from build123d import *

# Parameters (mm, degrees)
SKETCH1_W                    = 42.3
SKETCH1_H                    = 42.3
BOSS_EXTRUDE1_DEPTH          = 48
SKETCH2_R                    = 11
BOSS_EXTRUDE2_DEPTH          = 2
SKETCH3_R                    = 2.5
BOSS_EXTRUDE3_DEPTH          = 23
FILLET2_R                    = 0.3
CHAMFER1_SIZE                = 0.5
SKETCH4_R                    = 1.5
CUT_EXTRUDE1_DEPTH           = 4.5
CHAMFER2_SIZE                = 0.3
CUT_EXTRUDE2_START           = -0.5
SKETCH5_R                    = 16.5
SKETCH5_R_2                  = 11
CUT_EXTRUDE2_DEPTH           = 0.5
CUT_EXTRUDE_THIN1_DEPTH      = 57.556564606
CUT_EXTRUDE_THIN1_DEPTH_BACK = 57.556564606
SKETCH7_R                    = 3.5
SKETCH7_R_2                  = 3
CUT_EXTRUDE3_DEPTH           = 5
SKETCH8_W                    = 8
SKETCH8_H                    = 5
BOSS_EXTRUDE4_DEPTH          = 2
FILLET3_R                    = 1


with BuildPart() as part:
    # Sketch1 → Boss-Extrude1 (new body)
    with BuildSketch(Plane(origin=(0, 0, 0), x_dir=(1, 0, 0), z_dir=(0, 1, 0))):
        Rectangle(SKETCH1_W, SKETCH1_H)
    extrude(amount=BOSS_EXTRUDE1_DEPTH)

    # Sketch2 → Boss-Extrude2 (add)
    with BuildSketch(Plane(origin=(0, 48, 0), x_dir=(1, 0, 0), z_dir=(0, 1, 0))):
        with Locations(Location((0, 0, 0), (0, 0, 90))):
            Circle(SKETCH2_R)
    extrude(amount=BOSS_EXTRUDE2_DEPTH)

    # Sketch3 → Boss-Extrude3 (add)
    with BuildSketch(Plane(origin=(0, 50, 0), x_dir=(1, 0, 0), z_dir=(0, 1, 0))):
        with Locations(Location((0, 0, 0), (0, 0, 270))):
            Circle(SKETCH3_R)
    extrude(amount=BOSS_EXTRUDE3_DEPTH)

    # Fillet2
    fillet2_edges = [part.edges().sort_by_distance(p)[0] for p in [
        (0, 50, 11),
    ]]
    fillet(fillet2_edges, radius=FILLET2_R)

    # Chamfer1
    chamfer1_edges = [part.edges().sort_by_distance(p)[0] for p in [
        (0, 73, -2.5),
    ]]
    chamfer(chamfer1_edges, length=CHAMFER1_SIZE)

    # Sketch4 → Cut-Extrude1 (cut)
    with BuildSketch(Plane(origin=(0, 48, 0), x_dir=(1, 0, 0), z_dir=(0, 1, 0))):
        with Locations(Location((-15.5, -15.5, 0), (0, 0, 270))):
            Circle(SKETCH4_R)
        with Locations(Location((15.5, -15.5, 0), (0, 0, 270))):
            Circle(SKETCH4_R)
        with Locations(Location((15.5, 15.5, 0), (0, 0, 270))):
            Circle(SKETCH4_R)
        with Locations(Location((-15.5, 15.5, 0), (0, 0, 270))):
            Circle(SKETCH4_R)
    extrude(amount=-CUT_EXTRUDE1_DEPTH, mode=Mode.SUBTRACT)

    # Chamfer2
    chamfer2_edges = [part.edges().sort_by_distance(p)[0] for p in [
        (-15.5, 48, 14),
        (15.5, 48, 14),
        (15.5, 48, -17),
        (-15.5, 48, -17),
    ]]
    chamfer(chamfer2_edges, length=CHAMFER2_SIZE)

    # Sketch5 → Cut-Extrude2 (cut)
    with BuildSketch(Plane(origin=(0, 48, 0), x_dir=(1, 0, 0), z_dir=(0, 1, 0)).offset(CUT_EXTRUDE2_START)):
        with Locations(Location((0, 0, 0), (0, 0, 270))):
            Circle(SKETCH5_R)
        with Locations(Location((0, 0, 0), (0, 0, 270))):
            Circle(SKETCH5_R_2, mode=Mode.SUBTRACT)
    extrude(amount=CUT_EXTRUDE2_DEPTH, mode=Mode.SUBTRACT)

    # Sketch6 → Cut-Extrude-Thin1 (cut, two sides: drawn at the far end of the back side and taken through both)
    with BuildSketch(Plane(origin=(0, 48, 0), x_dir=(1, 0, 0), z_dir=(0, 1, 0)).offset(-CUT_EXTRUDE_THIN1_DEPTH_BACK)):
        Polygon((-21.15, -17.15), (-17.15, -21.15), (-24.221067812, -28.221067812), (-28.221067812, -24.221067812), align=None)
        Polygon((17.15, -21.15), (21.15, -17.15), (28.221067812, -24.221067812), (24.221067812, -28.221067812), align=None)
        Polygon((21.15, 17.15), (17.15, 21.15), (24.221067812, 28.221067812), (28.221067812, 24.221067812), align=None)
        Polygon((-17.15, 21.15), (-21.15, 17.15), (-28.221067812, 24.221067812), (-24.221067812, 28.221067812), align=None)
    extrude(amount=CUT_EXTRUDE_THIN1_DEPTH + CUT_EXTRUDE_THIN1_DEPTH_BACK, mode=Mode.SUBTRACT)

    # Sketch7 → Cut-Extrude3 (cut)
    with BuildSketch(Plane.XZ):
        with Locations(Location((0, 0, 0), (0, 0, 270))):
            Circle(SKETCH7_R)
        with Locations(Location((-15.5, 15.5, 0), (0, 0, 270))):
            Circle(SKETCH7_R_2)
        with Locations(Location((15.5, 15.5, 0), (0, 0, 270))):
            Circle(SKETCH7_R_2)
        with Locations(Location((15.5, -15.5, 0), (0, 0, 270))):
            Circle(SKETCH7_R_2)
        with Locations(Location((-15.5, -15.5, 0), (0, 0, 270))):
            Circle(SKETCH7_R_2)
    extrude(amount=-CUT_EXTRUDE3_DEPTH, mode=Mode.SUBTRACT)

    # Sketch8 → Boss-Extrude4 (add)
    with BuildSketch(Plane.ZY.offset(21.15)):
        with Locations((0, 5)):
            Rectangle(SKETCH8_W, SKETCH8_H)
    extrude(amount=BOSS_EXTRUDE4_DEPTH)

    # Fillet3
    fillet3_edges = [part.edges().sort_by_distance(p)[0] for p in [
        (-23.15, 5, 4),
        (-23.15, 7.5, 0),
        (-23.15, 5, -4),
        (-23.15, 2.5, 0),
    ]]
    fillet(fillet3_edges, radius=FILLET3_R)


solid = part.part
Can you work these out from the model? Positions are in its coordinate system, mm. A direction names the side the tool comes from. Give positions to 0.01 mm unless a question says otherwise; leave off trailing zeros. Write each loop counter-clockwise with the first axis right and the second up, starting at its lowest first coordinate (ties: lowest second). Pieces come first, ordered by that corner, then holes. Notation, with made-up numbers: (62.25, 39) -> (68.25, 39) arc R9 ccw to (68.25, 51) -> close; hole circle Ø8 at (43.5, -18). An arc over 180 degrees is marked (long way). Answer as a JSON object with one key per item and string values. Group by question number.
Item 1: Suppose I cut it at C-C (y = 46). Please give me the cut outline in (x, z).
Item 2: Suppose I cut it at A-A (x = 0). Please give me the cut outline in (y, z), plus the area to 3 significant figures.
Item 3: I'm going to push flat-ended pins straight in: P1, Ø10, axis at y = 37, z = 16, coming from the -X side; P2, Ø3.5, axis at x = 15.5, z = 15.5, coming from the +Y side; P3, Ø0.5, axis at x = -21.5, y = 4, coming from the +Z side; P4, Ø6, axis at x = -9, z = 6.5, coming from the -Y side. Where does each tip first touch, or does it pass through?
Item 4: For faces 1 (the face through (-3.417, 2.465, 0.759)), 2 (the face through (15.57, 45.63, 14)), 3 (the face through (-5, 0, 0)), which set-ups out of +Z, -Z, +X, -X, +Y, -Y let a thin tool reach every point of the face, with its end or its side?
Item 5: We'd pull the mould along X, two halves only. Please class faces 4 (the face through (-15.43, 45.63, 14)), 5 (the face through (-23.15, 5, 0)), 6 (the face through (21.15, 24, 0)): +X half, -X half, draft (parallel to the pull), parting line (faces both ways), or undercut.
Item 6: Please list where these lines run through material, in increasing order: line 1 (X direction, y = 2.3, z = -15.5); line 2 (Z direction, x = -15, y = 46); line 3 (Y direction, x = -17, z = 19). Write a range as [from, to].
Item 7: Suppose I cut it at D-D (y = 34.5). Please give me the cut outline in (x, z), plus the area to 3 significant figures.
Findings:
{
 "1": {"outline": "(-21.15, -17.15) -> (-17.15, -21.15) -> (17.15, -21.15) -> (21.15, -17.15) -> (21.15, 17.15) -> (17.15, 21.15) -> (-17.15, 21.15) -> (-21.15, 17.15) -> close; hole circle Ø3 at (-15.5, -15.5); hole circle Ø3 at (-15.5, 15.5); hole circle Ø3 at (15.5, -15.5); hole circle Ø3 at (15.5, 15.5)"},
 "2": {"outline": "(0, -21.15) -> (48, -21.15) -> (48, -16.5) -> (47.5, -16.5) -> (47.5, -11) -> (49.7, -11) arc R0.3 ccw to (50, -10.7) -> (50, -2.5) -> (72.5, -2.5) -> (73, -2) -> (73, 2) -> (72.5, 2.5) -> (50, 2.5) -> (50, 10.7) arc R0.3 ccw to (49.7, 11) -> (47.5, 11) -> (47.5, 16.5) -> (48, 16.5) -> (48, 21.15) -> (0, 21.15) -> (0, 3.5) -> (5, 3.5) -> (5, -3.5) -> (0, -3.5) -> close", "area": "2,150 mm²"},
 "3": {"P1": "stops at x = -21.15", "P2": "stops at y = 47.95", "P3": "stops at z = 4", "P4": "stops at y = 0"},
 "4": {"face 1": "-Y", "face 2": "+Y", "face 3": "+Z, -Z, +X, -X, -Y"},
 "5": {"face 4": "undercut", "face 5": "-X half", "face 6": "+X half"},
 "6": {"line 1": "x = [-21.15, -18.5], [-12.5, 12.5], [18.5, 21.15]", "line 2": "z = [-21.15, -16.91], [-14.09, 14.09], [16.91, 21.15]", "line 3": "y = [0, 48]"},
 "7": {"outline": "(-21.15, -17.15) -> (-17.15, -21.15) -> (17.15, -21.15) -> (21.15, -17.15) -> (21.15, 17.15) -> (17.15, 21.15) -> (-17.15, 21.15) -> (-21.15, 17.15) -> close", "area": "1,760 mm²"}
}
